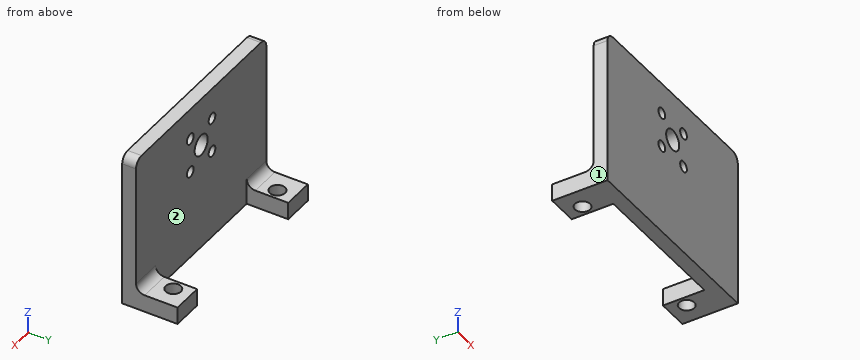
from build123d import *

# Parameters (mm, degrees)
SKETCH1_W           = 60
SKETCH1_H           = 4
BOSS_EXTRUDE1_DEPTH = 45
SKETCH1_3_R         = 2.2
BOSS_EXTRUDE2_DEPTH = 5
SKETCH2_R           = 3
SKETCH2_R_2         = 1.55
CUT_EXTRUDE1_DEPTH  = 5
BOSS_EXTRUDE3_DEPTH = 45
FILLET1_R           = 2.5
FILLET3_R           = 2.5
SKETCH3_R           = 4
BOSS_EXTRUDE4_DEPTH = 12
SKETCH4_R           = 6
BOSS_EXTRUDE5_DEPTH = 5
FILLET4_R           = 1
SKETCH5_W           = 46.619734532
SKETCH5_H           = 29.432499903
CUT_EXTRUDE3_DEPTH  = 61


with BuildPart() as part:
    # Sketch1 → Boss-Extrude1 (new body)
    with BuildSketch(Plane.XY):
        with Locations((-82.025641026, 5.685176195)):
            Rectangle(SKETCH1_W, SKETCH1_H)
    extrude(amount=BOSS_EXTRUDE1_DEPTH)

    # Sketch1_3 → Boss-Extrude2 (add)
    with BuildSketch(Plane.XY):
        Polygon((-112.025641026, 27.185176195), (-112.025641026, 7.685176195), (-103.025641026, 7.685176195), (-103.025641026, 27.185176195), (-103.025641026, 31.685176195), (-112.025641026, 31.685176195), align=None)
        with Locations((-106.025641026, 14.685176195)):
            Circle(SKETCH1_3_R, mode=Mode.SUBTRACT)
        with Locations((-106.025641026, 24.685176195)):
            Circle(SKETCH1_3_R, mode=Mode.SUBTRACT)
        Polygon((-61.025641026, 27.185176195), (-61.025641026, 7.685176195), (-52.025641026, 7.685176195), (-52.025641026, 27.185176195), (-52.025641026, 31.685176195), (-61.025641026, 31.685176195), align=None)
        with Locations((-58.025641026, 14.685176195)):
            Circle(SKETCH1_3_R, mode=Mode.SUBTRACT)
        with Locations((-58.025641026, 24.685176195)):
            Circle(SKETCH1_3_R, mode=Mode.SUBTRACT)
    extrude(amount=BOSS_EXTRUDE2_DEPTH)

    # Sketch2 → Cut-Extrude1 (cut, through all)
    with BuildSketch(Plane(origin=(0, 7.685176195, 0), x_dir=(1, 0, 0), z_dir=(0, 1, 0))):
        with Locations((-82.025641026, -31)):
            Circle(SKETCH2_R)
        with Locations((-77.025641026, -26)):
            Circle(SKETCH2_R_2)
        with Locations((-87.025641026, -26)):
            Circle(SKETCH2_R_2)
        with Locations((-77.025641026, -36)):
            Circle(SKETCH2_R_2)
        with Locations((-87.025641026, -36)):
            Circle(SKETCH2_R_2)
    extrude(amount=-CUT_EXTRUDE1_DEPTH, mode=Mode.SUBTRACT)

    # Sketch1_4 → Boss-Extrude3 (add)
    with BuildSketch(Plane.XY):
        Polygon((-112.025641026, 35.685176195), (-112.025641026, 31.685176195), (-103.025641026, 31.685176195), (-61.025641026, 31.685176195), (-52.025641026, 31.685176195), (-52.025641026, 35.685176195), align=None)
    extrude(amount=BOSS_EXTRUDE3_DEPTH)

    # Fillet1
    fillet1_edges = [part.edges().sort_by_distance(p)[0] for p in [
        (-112.025641026, 5.685176195, 45),
        (-52.025641026, 5.685176195, 45),
        (-112.025641026, 33.685176195, 45),
        (-52.025641026, 33.685176195, 45),
    ]]
    fillet(fillet1_edges, radius=FILLET1_R)

    # Fillet3
    fillet3_edges = [part.edges().sort_by_distance(p)[0] for p in [
        (-107.525641026, 31.685176195, 5),
        (-107.525641026, 7.685176195, 5),
        (-56.525641026, 31.685176195, 5),
        (-56.525641026, 7.685176195, 5),
    ]]
    fillet(fillet3_edges, radius=FILLET3_R)

    # Sketch3 → Boss-Extrude4 (add)
    with BuildSketch(Plane(origin=(0, 35.685176195, 0), x_dir=(1, 0, 0), z_dir=(0, 1, 0))):
        with Locations((-82.025641026, -31)):
            Circle(SKETCH3_R)
    extrude(amount=BOSS_EXTRUDE4_DEPTH)

    # Sketch4 → Boss-Extrude5 (add)
    with BuildSketch(Plane(origin=(0, 35.685176195, 0), x_dir=(1, 0, 0), z_dir=(0, 1, 0))):
        with Locations((-82.025641026, -31)):
            Circle(SKETCH4_R)
    extrude(amount=BOSS_EXTRUDE5_DEPTH)

    # Fillet4
    fillet4_edges = [part.edges().sort_by_distance(p)[0] for p in [
        (-86.025641026, 40.685176195, 31),
    ]]
    fillet(fillet4_edges, radius=FILLET4_R)

    # Sketch5 → Cut-Extrude3 (cut, through all)
    with BuildSketch(Plane.ZY.offset(112.025641026)):
        with Locations((23.309867266, 34.401426147)):
            Rectangle(SKETCH5_W, SKETCH5_H)
    extrude(amount=-CUT_EXTRUDE3_DEPTH, mode=Mode.SUBTRACT)


solid = part.part
Can you work these out from the model? Positions are in its coordinate system, mm. Face numbers are marked on the shaded views. A direction names the side the tool comes from. Coordinates: 2 decimals unless noted, no trailing zeros. Loops run counter-clockwise (first coordinate to the right, second up) from the corner with the lowest first, then second, coordinate; pieces in that order, holes last. Notation, with made-up numbers: M 16,16 L 20,16 A26 ccw 20,36 Z; hole C -10,22 d8. An arc over 180 degrees is marked long. Return JSON: item names as keys, results as strings. Group by question number.
Item 1: Imagine slicing it at B-B (y = 18.75). Please give me the cut outline in (x, z), and give its area (3 significant figures).
Item 2: I'm going to push flat-ended pins straight in: pin 1 Ø2.5 at (x, y) = (-106.03, 14.69) entering from +Z; pin 2 Ø4 at (x, z) = (-87.03, 26) entering from +Y; pin 3 Ø4.5 at (x, y) = (-107.5, 14.5) entering from +Z. Where does each tip first touch, or does it pass through?
Item 3: Imagine slicing it at A-A (z = 36). Please give me the cut outline in (x, y), and give its area (3 significant figures).
Item 4: Imagine slicing it at C-C (z = 31). Please give me the cut outline in (x, y).
Item 5: If I drill on L1, parallel to X at y = 6.65, z = 26; L2, parallel to X at y = 6.3, z = 31; L3, parallel to Y at x = -99, z = 35, over which ranges is the centre line in solid material (lowest first)? Write a range as from..to.
Item 6: Imagine slicing it at D-D (x = -107). Please give me the cut outline in (y, z), and give its area (3 significant figures).
Item 7: On a 3-axis mill with a long thin cutter (end or side, diameter ignored), from which of +Z, -Z, +X, -X, +Y, -Y can I reach the whole of each face in a straight line? I mean the marked faces 1 and 2. Say none if no direction works.
Verdict:
{
 "1": {"outline": "M -112.03,0 L -103.03,0 L -103.03,5 L -112.03,5 Z; M -61.03,0 L -52.03,0 L -52.03,5 L -61.03,5 Z", "area": "90.0 mm^2"},
 "2": {"pin 1": "passes through", "pin 2": "stops at y = 7.69", "pin 3": "stops at z = 5"},
 "3": {"outline": "M -112.03,3.69 L -88.58,3.69 L -88.58,7.69 L -112.03,7.69 Z; M -85.48,3.69 L -78.58,3.69 L -78.58,7.69 L -85.48,7.69 Z; M -75.48,3.69 L -52.03,3.69 L -52.03,7.69 L -75.48,7.69 Z", "area": "215 mm^2"},
 "4": {"outline": "M -112.03,3.69 L -85.03,3.69 L -85.03,7.69 L -112.03,7.69 Z; M -79.03,3.69 L -52.03,3.69 L -52.03,7.69 L -79.03,7.69 Z"},
 "5": {"L1": "x = -112.03..-88.58, -85.48..-78.58, -75.48..-52.03", "L2": "x = -112.03..-85.03, -79.03..-52.03", "L3": "y = 3.69..7.69"},
 "6": {"outline": "M 3.69,0 L 12.71,0 L 12.71,5 L 10.19,5 A2.5 cw 7.69,7.5 L 7.69,45 L 3.69,45 Z; M 16.66,0 L 19.69,0 L 19.69,5 L 16.66,5 Z", "area": "222 mm^2"},
 "7": {"face 1": "+Z, -Z, -X, +Y, -Y", "face 2": "+Z, +Y"}
}
